Input: part model. Units: mm. Frame: model coordinates. Coordinates: 2 decimals unless noted, no trailing zeros. Write each loop counter-clockwise with the first axis right and the second up, starting at its lowest first coordinate (ties: lowest second). Pieces come first, ordered by that corner, then holes. Notation, with made-up numbers: (44.5, 14.5) - (67.5, 14.5) arc R12 ccw to (67.5, 18.5) - close; hole circle Ø3 at (13.5, -10.75). An arc over 180 degrees is marked (long way). Put each result on its own line as item: value. Start each with the question number.
1. Line query: line 1 (Z direction, x = -15, y = 8); line 2 (Z direction, x = -78.5, y = 3); line 3 (X direction, y = 7, z = -143.5). Output: solid intervals per line, ascending.
2. Cut plane B-B, the plane x = -62.5. Return loops of the section in (y, z).
3. Cut plane A-A, the plane y = 10. Return loops of the section in (x, z), and give its area (3 significant figures).
4. Pin query (flat end, axial travel): pin 1 (5 mm diameter, centred on y = 5.5, z = -151, fed in from -X); pin 2 (6 mm diameter, centred on x = -32.5, y = 3, fed in from -Z); pin 3 (1 mm diameter, centred on y = 4, z = -136, fed in from -X). Return the tip coordinate at first contact, or that it passes through.
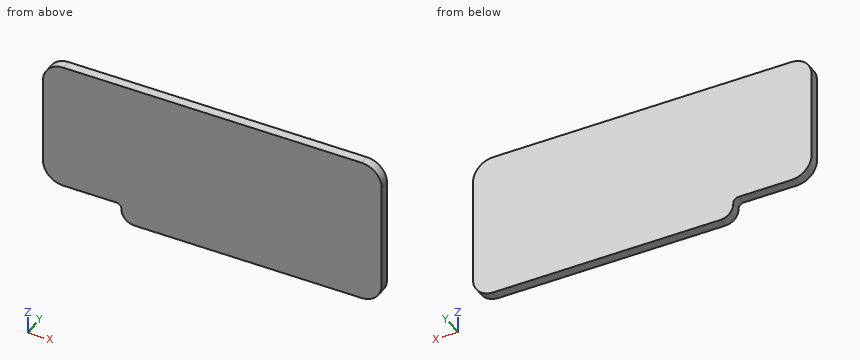
from build123d import *

# Parameters (mm, degrees)
EXTRUDE_1_DEPTH = 12


with BuildPart() as part:
    # Эскиз1 → Бобышка-Вытянуть1 (new body)
    with BuildSketch(Plane(origin=(0, 0, 0), x_dir=(1, 0, 0), z_dir=(0, 1, 0))):
        with BuildLine():
            Line((0, 0), (297, 0))
            ThreePointArc((297, 0), (314.67766953, 7.32233047), (322, 25))
            Line((322, 25), (322, 155))
            ThreePointArc((322, 155), (314.67766953, 172.67766953), (297, 180))
            Line((297, 180), (16, 180))
            ThreePointArc((16, 180), (4.686291501, 175.313708499), (0, 164))
            Line((0, 164), (0, 162.982))
            ThreePointArc((0, 162.982), (-1.757359313, 158.739359313), (-6, 156.982))
            Line((-6, 156.982), (-72, 156.982))
            ThreePointArc((-72, 156.982), (-89.67766953, 149.65966953), (-97, 131.982))
            Line((-97, 131.982), (-97, 25))
            ThreePointArc((-97, 25), (-89.67766953, 7.32233047), (-72, 0))
            Line((-72, 0), (0, 0))
        make_face()
    extrude(amount=EXTRUDE_1_DEPTH)


solid = part.part
Report:
1. line 1: z = -156.98 to 0
1. line 2: z = -156.12 to -0.86
1. line 3: x = -94.19 to 322
2. outline: (0, -156.98) - (12, -156.98) - (12, 0) - (0, 0) - close
3. outline: (-97, -131.98) arc R25 ccw to (-72, -156.98) - (-6, -156.98) arc R6 cw to (0, -162.98) - (0, -164) arc R16 ccw to (16, -180) - (297, -180) arc R25 ccw to (322, -155) - (322, -25) arc R25 ccw to (297, 0) - (-72, 0) arc R25 ccw to (-97, -25) - close
3. area: 72,600 mm^2
4. pin 1: stops at x = -90.77
4. pin 2: stops at z = -156.98
4. pin 3: stops at x = -96.75
